Design review of the part built by this model. Coordinates are the model's own, in mm. A direction names the side the tool comes from. Coordinates: 2 decimals unless noted, no trailing zeros. Write each loop counter-clockwise with the first axis right and the second up, starting at its lowest first coordinate (ties: lowest second). Pieces come first, ordered by that corner, then holes. Notation, with made-up numbers: (-0.75, 37) - (36.25, 37) arc R24 ccw to (36.25, 48) - close; hole circle Ø4 at (-36.75, 46). An arc over 180 degrees is marked (long way). Use a Markdown table: item, result.
Autodesk Inventor part; units mm, degrees
ref_plane "YZ Plane" through (0, 0, 0) normal (1, 0, 0) x (0, 1, 0)
ref_plane "XZ Plane" through (0, 0, 0) normal (0, 1, 0) x (-1, 0, 0)
ref_plane "XY Plane" through (0, 0, 0) normal (0, 0, 1) x (1, 0, 0)
sketch "Sketch1" plane through (0, 0, 0) normal (1, 0, 0) x (0, 1, 0)
  circle A0 centre (0, 0) radius 30
  circle A1 centre (0, 0) radius 30
  dimension "d0" = 60
  dimension "d22" = 60
extrude "Extrusion1" add sketch "Sketch1" along normal blind 10
sketch "Sketch2" plane through (10, 0, 0) normal (1, 0, 0) x (0, 0, -1)
  point P0 (0, 0)
  point P1 (-8, 8)
  point P2 (8, 8)
  point P3 (8, -8)
  point P4 (-8, -8)
  dimension "d3" = 8
  dimension "d4" = 8
  dimension "d5" = 16
  dimension "d6" = 16
hole "Hole1" at (10, 8, 8) at (10, 8, -8) at (10, -8, -8) at (10, -8, 8) direction (-1, 0, 0) diameter 5 end through all counterbore diameter 6 counterbore depth 2
sketch "Sketch3" plane through (10, 0, 0) normal (1, 0, 0) x (0, 0, -1)
  point P0 (0, 0)
  point P1 (0, 0)
hole "Hole2" at (10, 0, 0) direction (-1, 0, 0) diameter 8 end through all
equation "\"d0\" = d22"
properties part number "Tapon 1"
(1) Draft analysis for pull direction Y (two halves, no side actions). For faces 1 (the cylindrical face through (3.94, 10.22, -9.15)), 2 (the flat face through (10, 0, -6)), 3 (the cylindrical face through (4.93, -29.97, -1.32)), state which applies: +Y half, -Y half, draft (parallel to the pull), parting line (faces both ways), or undercut.
Determined:
| item | result |
|---|---|
| face 1 | undercut |
| face 2 | draft |
| face 3 | parting line |
(2) Take a section at A-A on z = 0. Write out the cut boundary in (x, y).
Determined:
| item | result |
|---|---|
| outline | (0, -30) - (10, -30) - (10, -4) - (0, -4) - close; (0, 4) - (10, 4) - (10, 30) - (0, 30) - close |
(3) For pin 1 (1 mm diameter, centred on x = 7.5, z = -7, fed in from -Y); pin 2 (2 mm diameter, centred on x = 6.5, y = 20.5, fed in from -Z); pin 3 (2 mm diameter, centred on x = 1, z = 13.5, fed in from +Y), all flat-tipped, find the tip position at first contact; note any pin that passes through.
Determined:
| item | result |
|---|---|
| pin 1 | y = -29.29 |
| pin 2 | z = -22.8 |
| pin 3 | y = 27.27 |
(4) Take a section at C-C on x = 3.5. Write out the cut boundary in (y, z).
Determined:
| item | result |
|---|---|
| outline | circle Ø60 at (0, 0); hole circle Ø5 at (-8, -8); hole circle Ø5 at (-8, 8); hole circle Ø8 at (0, 0); hole circle Ø5 at (8, -8); hole circle Ø5 at (8, 8) |
(5) For L1, parallel to Y at x = 4, z = 8; L2, parallel to Z at x = 8.65, y = -8, list the stretches that pass through material, from the lowest coordinate up. Write a range as from..to.
Determined:
| item | result |
|---|---|
| L1 | -28.91..-10.5, -5.5..5.5, 10.5..28.91 |
| L2 | -28.91..-11, -5..5, 11..28.91 |
(6) Take a section at B-B on y = -6.5. Write out the cut boundary in (x, z), and give its area (3 significant figures).
Determined:
| item | result |
|---|---|
| outline | (0, -29.29) - (10, -29.29) - (10, -10.6) - (8, -10.6) - (8, -10) - (0, -10) - close; (0, -6) - (8, -6) - (8, -5.4) - (10, -5.4) - (10, 5.4) - (8, 5.4) - (8, 6) - (0, 6) - close; (0, 10) - (8, 10) - (8, 10.6) - (10, 10.6) - (10, 29.29) - (0, 29.29) - close |
| area | 501 mm2 |
(7) Machinability: for faces 4 (the flat face through (8, -10, 10)), 5 (the cylindrical face through (4.93, 3.905, 0.867)), which of the approach directions +Z, -Z, +X, -X, +Y, -Y give a long, thin tool a straight path to every point of the face, cutting with its end or side? Answer none if there is none.
Determined:
| item | result |
|---|---|
| face 4 | +X |
| face 5 | +X, -X |
